from build123d import *

# Parameters (mm, degrees)
F0_W     = 254
F0_H     = 19.05
F1_DEPTH = 768.35
F2_SIZE2 = 19.04999
F2_SIZE  = 19.04999


# Not quite as in the source:
# - a fillet or chamfer is up to 0.001 mm smaller than in the source, because OpenCascade refuses the exact size


with BuildPart() as f1:
    # F0 (on Top) → F1 (new body, symmetric)
    with BuildSketch(Plane.XY):
        Rectangle(F0_W, F0_H)
    extrude(amount=F1_DEPTH, both=True)

    # F2 (size 19.05 and 19.05 in the source; OpenCascade refuses exactly that, so slightly less here)
    f2_edges = [f1.edges().sort_by_distance(p)[0] for p in [
        (0, 9.525, 768.35),
        (0, 9.525, -768.35),
    ]]
    chamfer(f2_edges, length=F2_SIZE, length2=F2_SIZE2)


solid = f1.part
Geometry: final body of the model. Coordinates: model frame, mm. Round coordinates to 2 decimals unless told otherwise and drop trailing zeros. Loops run counter-clockwise (first coordinate to the right, second up) from the corner with the lowest first, then second, coordinate; pieces in that order, holes last. Notation, with made-up numbers: M 20,82 L 35,82 A17 cw 35,108 Z; hole C -26.75,-24.75 d8. An arc over 180 degrees is marked long. Put each result on its own line as item: value. Start each with the question number.
(1) Section query A-A (y = 5.25). Return loops of the section in (x, z).
(2) Material intervals for line 1 along Z through (x, y) = (76, -8.25) (3 decimals); line 2 along Z through (x, y) = (-40, 4.5) (3 decimals), sorted ascending. Write a range as [from, to].
(3) Contact query for flat-ended pins moving along their axis: pin 1 Ø6 at (x, y) = (-90.5, 3.5) entering from -Z (3 decimals); pin 2 Ø3 at (x, y) = (80.5, 4) entering from +Z (3 decimals); pin 3 Ø4 at (x, y) = (0, -4) entering from +Z (3 decimals). Output: stop coordinate, or through.
Findings below:
1. outline: M -127,-753.58 L 127,-753.58 L 127,753.58 L -127,753.58 Z
2. line 1: z = [-767.075, 767.075]
2. line 2: z = [-754.325, 754.325]
3. pin 1: stops at z = -758.325
3. pin 2: stops at z = 756.325
3. pin 3: stops at z = 764.825
